Part model, mm, in its own coordinate system. A direction names the side the tool comes from. Coordinates: 2 decimals unless noted, no trailing zeros. Loops run counter-clockwise (first coordinate to the right, second up) from the corner with the lowest first, then second, coordinate; pieces in that order, holes last. Notation, with made-up numbers: M 63.5,73 L 76.5,73 A8 cw 76.5,86 Z; hole C 45.5,66 d3. An arc over 180 degrees is marked long. Answer as a JSON object with one key per item and string values. Group by question number.
1. Saw through at C-C on y = 4. Write the cut outline in (x, z).
2. Mould opens along X. For faces 1 (the face through (-16.1, -8.5, -15)), 2 (the face through (-6.08, -4.16, -10.11)), 3 (the face through (-9, -9, -29.288)), 4 (the face through (-2, 0.375, -19)) say: released by +X, released by -X, zero draft, split by the parting line, or undercut.
3. 3-axis set-ups, long thin cutter, end or side, ignore diameter. For faces 5 (the face through (-14, -12, -25.732)), 6 (the face through (-8, 4.477, -15)), 7 (the face through (-6.08, -4.16, -19.61)), 8 (the face through (-10, 8, -2.774)): which of +Z, -Z, +X, -X, +Y, -Y reach the whole face in a straight line?
4. Saw through at D-D on y = -14. Write the cut outline in (x, z) (1 decimal), then the cut area to 3 significant figures.
5. Saw through at B-B on x = -3.5. Count the separate pieces of the cut face and the enclosed holes in it, then the cut area to 3 significant figures.
6. Drop flat-ended pins along their axis: pin 1 Ø2 at (x, z) = (-4.5, -10.5) entering from +Y; pin 2 Ø0.9 at (y, z) = (4, -13.5) entering from -X; pin 3 Ø3 at (y, z) = (-13.5, -15) entering from +X; pin 4 Ø2.5 at (x, z) = (-3.581, -10) entering from +Y. Give the stop position or say it passes through.
7. Drill centre lines: L1, parallel to X at y = 6, z = -20.75; L2, parallel to Z at x = -4.5, y = 4; L3, parallel to Z at x = -7, y = -2. Where is each one in solid material? Low to high.
Autodesk Inventor part; units mm, degrees
ref_plane "Work Plane1" through (-11.25, 0, 0) normal (0, 0, 1) x (1, 0, 0)
ref_plane "YZ Plane" through (0, 0, 0) normal (1, 0, 0) x (0, 1, 0)
ref_plane "XZ Plane" through (0, 0, 0) normal (0, 1, 0) x (-1, 0, 0)
sketch "Sketch1" plane through (0, 0, 0) normal (0, 1, 0) x (-1, 0, 0)
  line L0 (0, 0) -> (15, 0)
  line L1 (15, 0) -> (15, -29.5)
  line L2 (15, -29.5) -> (0, -29.5)
  line L3 (0, -29.5) -> (0, 0)
  dimension "d0" = 15
  dimension "d1" = 29.5
extrude "Extrusion1" add sketch "Sketch1" along normal blind 5
fillet "Fillet1" radius 5 2 edges at (-7.5, 5, 0) (-7.5, 5, -29.5)
sketch "Sketch2" plane through (0, 0, 0) normal (0, -1, 0) x (1, 0, 0)
  circle A0 centre (-3.581, -10) radius 1.5
  line L0 (-15, -29.5) -> (-15, 0)
  line L1 (-15, -14.75) -> (-4.074, -14.75)
  line L2 (-4.074, 0) -> (-4.074, -29.5)
  circle A1 centre (-3.581, -19.5) radius 1.5
  line L3 (0, -27.3987) -> (0, -2.1013)
  point P0 (0, 0)
  dimension "d6" = 3
  dimension "d7" = 4.75
  dimension "d8" = 10.926
  dimension "d10" = 3
  dimension "d11" = 4.75
  dimension "d15" = 3.581
  dimension "d16" = 3.581
extrude "Extrusion2" cut sketch "Sketch2" against normal up to surface (5 mm away)
fillet "Fillet3" radius 1.993 1 edges at (-15, 0, -14.75)
sketch "Sketch3" plane through (0, 0, 0) normal (0, -1, 0) x (1, 0, 0)
  circle A0 centre (-3.581, -10) radius 2.5
  circle A1 centre (-3.581, -19.5) radius 2.5
  circle A2 centre (-3.581, -10) radius 1.5
  circle A3 centre (-3.581, -19.5) radius 1.5
  point P0 (0, 0)
  dimension "d18" = 5
  dimension "d19" = 5
  dimension "d20" = 0
  dimension "d21" = 0
  dimension "d22" = 0
  dimension "d23" = 0
extrude "Extrusion3" cut sketch "Sketch3" along normal blind 32.5 and the other way blind 0.375
sketch "Sketch4" plane through (-15, 5, -24.5) normal (-1, 0, 0) x (0, 0, 1)
  line L0 (24.5, -3.007) -> (-5, -3.007)
  line L1 (-5, -3.007) -> (-5, 0)
  line L2 (-5, 0) -> (24.5, 0)
  line L3 (24.5, 0) -> (24.5, -3.007)
  line L4 (-5, -5) -> (24.5, -5)
  line L5 (0, 0) -> (19.5, 0)
  dimension "d26" = 1.993
  dimension "d27" = 0
  dimension "d28" = 0
  dimension "d29" = 0
extrude "Extrusion4" add sketch "Sketch4" against normal blind 4.356
sketch "Sketch6" plane through (-15, 1.993, -29.5) normal (0, 0, -1) x (-1, 0, 0)
  line L0 (-3.661, 2.484) -> (-3.051, 2.484)
  line L1 (-0.856, 2.484) -> (-0.856, 8.484)
  line L2 (-0.856, 8.484) -> (-5.856, 8.484)
  line L3 (-5.856, 8.484) -> (-5.856, 2.484)
  line L4 (-15, -1.993) -> (-1.993, -1.993)
  line L5 (0, 3.007) -> (0, 0)
  line L6 (-15, -1.993) -> (-15, 3.007)
  line L7 (-4.356, 8.484) -> (-4.356, 3.179)
  line L8 (-2.356, 8.484) -> (-2.356, 3.179)
  arc A0 (-4.356, 3.179) -> (-3.661, 2.484) centre (-3.661, 3.179) ccw
  arc A1 (-3.051, 2.484) -> (-2.356, 3.179) centre (-3.051, 3.179) ccw
  line L9 (-0.856, 2.484) -> (-3.051, 2.484)
  line L10 (-5.856, 2.484) -> (-3.661, 2.484)
  line L11 (-5.856, 2.484) -> (-7.856, 2.484)
  line L12 (-15, 3.007) -> (-4.356, 3.007)
  line L13 (-5.856, 2.484) -> (-3.856, 2.484) construction
  line L14 (-7.856, 2.484) -> (-7.856, 8.484)
  line L15 (-7.856, 3.3104) -> (-5.856, 3.3104)
  point P0 (-10.926, -1.993)
  point P1 (-4.356, -1.993)
  dimension "d37" = 4.477
  dimension "d38" = 0.856
  dimension "d39" = 10.477
  dimension "d40" = 9.144
  dimension "d41" = 1.5
  dimension "d42" = 1.5
  dimension "d43" = 2
  dimension "d44" = 0.695
  dimension "d45" = 2
  dimension "d46" = 180
extrude "Extrusion6" cut sketch "Sketch6" against normal up to surface (29.5 mm away)
extrude "Extrusion7" add sketch "Sketch6" against normal up to surface (29.5 mm away) contours L10 L3 L2 L7 A0 | A1 L8 L2 L1 L9
extrude "Extrusion8" cut sketch "Sketch6" against normal blind 2.774 contours L10 L3 L2 L7 A0 | A1 L8 L2 L1 L9
sketch "Sketch7" plane through (-15, 1.993, 0) normal (0, 0, 1) x (1, 0, 0)
  line L0 (5.856, 8.484) -> (5.856, 2.484)
  line L1 (5.856, 2.484) -> (0.856, 2.484)
  line L2 (0.856, 2.484) -> (0.856, 11.6469)
  line L3 (0.856, 11.6469) -> (5.856, 11.6469)
  line L4 (5.856, 11.6469) -> (5.856, 2.484)
  line L5 (0.856, 3.007) -> (0.856, 8.484)
  point P0 (15, -1.993)
  dimension "d53" = 0
extrude "Extrusion9" cut sketch "Sketch7" against normal blind 2.774
sketch "Sketch8" plane through (-10.644, 5, -24.5) normal (1, 0, 0) x (0, 0, -1)
  arc A0 (4.5856, -3.007) -> (2.2263, -0.523) centre (0, -5) ccw
  arc A1 (4.5856, -3.007) -> (2.2263, -0.523) centre (0, -5) ccw
  line L0 (4.5856, -3.007) -> (5, -3.007)
  line L1 (4.5856, -3.007) -> (5, -3.007)
  line L2 (5, -3.007) -> (5, -0.523)
  line L3 (5, -3.007) -> (5, -0.523)
  line L4 (-24.5, 0) -> (5, 0)
  line L5 (5, -0.523) -> (5, 0)
  line L6 (5, 0) -> (2.226, 0)
  line L7 (2.226, -0.523) -> (2.226, 5.477)
  line L8 (2.226, -0.523) -> (2.226, 0)
  arc A2 (-19.5, 0) -> (-24.5, -5) centre (-19.5, -5) ccw
  line L9 (-24.0856, -3.007) -> (4.5856, -3.007)
  arc A3 (-21.7263, -0.523) -> (-24.0856, -3.007) centre (-19.5, -5) ccw
  line L10 (-24.5, -3.007) -> (-24.0856, -3.007)
  line L11 (-24.0856, -3.007) -> (-24.5, -3.007)
  line L12 (-24.5, -3.007) -> (-24.5, 0)
  line L13 (-24.5, 0) -> (-21.7263, 0)
  line L14 (2.2263, -0.523) -> (-21.7263, -0.523)
  line L15 (-21.7263, -0.523) -> (-21.7263, 0)
  line L16 (-21.726, 5.477) -> (-21.726, -0.523)
  point P0 (-22.3987, -0.926)
  point P1 (-24.0856, -3.007)
  point P2 (2.226, 0)
extrude "Extrusion10" cut sketch "Sketch8" against normal blind 9.726 contours A0 L7 L4 L5 L2 L0 | L10 L12 L4 L15 A2
ref_plane "Work Plane1" through (-11.25, 0, 0) normal (0, 0, 1) x (1, 0, 0)
sketch "Sketch9" plane through (-11.25, 0, 0) normal (0, 0, 1) x (1, 0, 0)
  line L0 (11.25, 0) -> (-1.757, 0)
  line L1 (11.25, 0) -> (17.6322, 0) construction
  line L2 (11.25, 0) -> (6.4097, 2.5736)
  line L3 (6.4097, 2.5736) -> (-5.3271, -19.5)
  line L4 (-5.3271, -19.5) -> (-0.4868, -22.0737)
  line L5 (-0.4868, -22.0737) -> (11.25, 0)
  line L6 (11.25, 0) -> (15.8244, 0)
  point P0 (5.0413, 0)
  dimension "d59" = 5.482
  dimension "d60" = 25
  dimension "d61" = 118
  dimension "d62" = 0
  dimension "d63" = 0
extrude "Extrusion11" add sketch "Sketch9" against normal blind 29.5 contours L5 L4 L3 L0
sketch "Sketch10" plane through (-16.5771, -19.5, -29.5) normal (-0.4694716, -0.8829476, 0) x (0.8829476, -0.4694716, 0)
  line L0 (5.482, 29.2875) -> (0, 29.2875)
  line L1 (0, 29.2875) -> (0, 0.2125)
  line L2 (0, 0.2125) -> (5.482, 0.2125)
  line L3 (5.482, 0.2125) -> (5.482, 29.2875)
  line L4 (5.482, 29.5) -> (5.482, 0)
  line L5 (0, 29.5) -> (0, 0)
  line L6 (5.482, 0) -> (0, 0)
  line L7 (0, 29.5) -> (5.482, 29.5)
  point P0 (5.482, 0.2125)
  point P1 (0, 0.2125)
  point P2 (0, 29.2875)
  point P3 (5.482, 29.2875)
  dimension "d66" = 0
  dimension "d67" = 0
  dimension "d68" = 0.2125
  dimension "d69" = 0.2125
  dimension "d70" = 29.075
extrude "Extrusion12" cut sketch "Sketch10" against normal up to surface contours L0 L5 L7 L4 | L4 L6 L5 L2 surface through (-7.5, 0, -14.75) normal (0, 1, 0)
sketch "Sketch11" plane through (-11.7368, -22.0737, -29.2875) normal (-0.4694716, -0.8829476, 0) x (0.8829476, -0.4694716, 0)
  line L0 (-5.482, 0) -> (-5.482, 29.075)
  line L1 (0, 0) -> (-5.482, 0)
  line L2 (-5.482, 29.075) -> (-5.382, 29.075)
  line L3 (-5.382, 29.075) -> (-5.382, 0)
  line L4 (-5.382, 0) -> (-5.482, 0)
  line L5 (-5.482, 0) -> (-5.482, 29.075)
  point P0 (0, 29.2875)
  dimension "d73" = 0.1
extrude "Extrusion13" cut sketch "Sketch11" against normal up to surface surface through (-7.5, 0, -14.75) normal (0, 1, 0)
sketch "Sketch12" plane through (-16.4888, -19.547, -29.2875) normal (-0.8829476, 0.4694716, 0) x (0, 0, 1)
  line L0 (25.519, 0) -> (3.556, 0)
  line L1 (3.556, 0) -> (3.556, 17.1383)
  line L2 (3.556, 17.1383) -> (25.519, 17.1383)
  line L3 (25.519, 17.1383) -> (25.519, 0)
  line L4 (29.075, 0) -> (0, 0)
  line L5 (0, 0) -> (0, 22.1383)
  line L6 (0, 22.1383) -> (29.075, 22.1383)
  line L7 (29.075, 22.1383) -> (29.075, 0)
  line L8 (29.075, 17.1383) -> (0, 17.1383)
  line L9 (0, 17.1383) -> (0, 22.1383)
  line L10 (0, 22.1383) -> (29.075, 22.1383)
  line L11 (29.075, 22.1383) -> (29.075, 17.1383)
  point P0 (29.2875, 25)
  point P1 (3.556, 17.1383)
  point P2 (25.519, 17.1383)
  dimension "d76" = 0
  dimension "d77" = 21.963
  dimension "d78" = 29.075
  dimension "d79" = 3.556
  dimension "d80" = 5
extrude "Extrusion14" add sketch "Sketch12" along normal blind 2.342 contours L0 L1 L2 L3 | L2 L8 L5 L6 L7
sketch "Sketch13" plane through (-18.5567, -18.4475, -29.2875) normal (-0.8829476, 0.4694716, 0) x (0, 0, 1)
  line L0 (0, 20.8931) -> (29.075, 20.8931)
  line L1 (29.075, 0) -> (0, 0)
  line L2 (0, 0) -> (0, 20.8931)
  line L3 (0, 20.8931) -> (29.075, 20.8931)
  line L4 (29.075, 20.8931) -> (29.075, 0)
  point P0 (29.2875, 25)
  point P1 (29.075, 20.8931)
extrude "Extrusion15" add sketch "Sketch13" along normal blind 2.5
sketch "Sketch14" plane through (-11.7368, -22.0737, -29.2875) normal (-0.4694716, -0.8829476, 0) x (0.8829476, -0.4694716, 0)
  line L0 (0, 16.5425) -> (-2.05, 16.5425)
  line L1 (-2.05, 16.5425) -> (-2.05, 12.5325)
  line L2 (-2.05, 12.5325) -> (0, 12.5325)
  line L3 (0, 12.5325) -> (0, 16.5425)
  line L4 (0, 29.075) -> (0, 0)
  line L5 (-5.382, 0) -> (0, 0)
  point P0 (0, 29.2875)
  dimension "d85" = 0
  dimension "d86" = 4.01
  dimension "d87" = 29.075
  dimension "d88" = 12.5325
  dimension "d89" = 2.05
extrude "Extrusion16" cut sketch "Sketch14" against normal blind 20
extrude "Extrusion17" cut sketch "Sketch3" along normal blind 32.5 contours A0 | A1 | A2 | A3
properties part number "bottomclip"
Outcome:
{
 "1": {"outline": "M -15,-27.5 L 0,-27.5 L 0,-2 L -15,-2 Z; hole C -3.58,-19.5 d3; hole C -3.58,-10 d3"},
 "2": {"face 1": "released by -X", "face 2": "undercut", "face 3": "zero draft", "face 4": "undercut"},
 "3": {"face 5": "-Z", "face 6": "+Z, -Z, +Y", "face 7": "-Y", "face 8": "+Z, +X, -X, +Y"},
 "4": {"outline": "M -19,-29.3 L -16.2,-29.3 L -16.2,-25.7 L -13.5,-25.7 L -13.5,-29.3 L -7.4,-29.3 L -7.4,-16.8 L -9.8,-16.8 L -9.8,-12.7 L -7.4,-12.7 L -7.4,-0.2 L -13.5,-0.2 L -13.5,-3.8 L -16.2,-3.8 L -16.2,-0.2 L -19,-0.2 Z", "area": "308 mm²"},
 "5": {"separate pieces": "3", "enclosed holes": "0", "area": "220 mm²"},
 "6": {"pin 1": "stops at y = 5", "pin 2": "stops at x = -15", "pin 3": "stops at x = -8.7", "pin 4": "passes through"},
 "7": {"L1": "x = -14.14 to -12.64, -10.64 to -9.14", "L2": "z = -27.5 to -20.69, -18.31 to -11.19, -8.81 to -2", "L3": "z = -29.29 to -0.21"}
}
